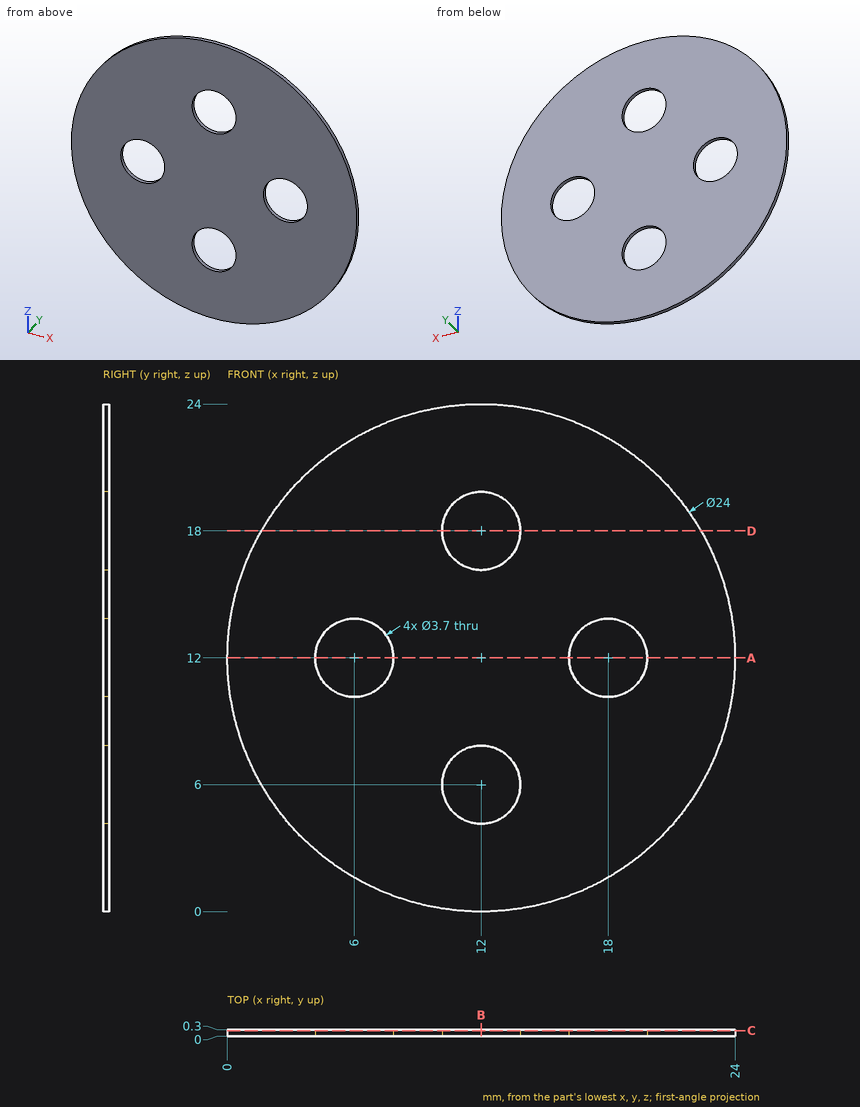
Answer from the drawing. Dimensions are ordinates in mm from the lowest x, y and z of the part. Round coordinates to 2 decimals unless told otherwise and drop trailing zeros. Write each loop counter-clockwise with the first axis right and the second up, starting at its lowest first coordinate (ties: lowest second). Pieces come first, ordered by that corner, then holes. Notation, with made-up numbers: (84.5, 13) - (129.5, 13) arc R32 cw to (129.5, 39) - close; hole circle Ø7 at (-18.75, -21.5). An arc over 180 degrees is marked (long way). One line per item, written item: value.
Q1. Find section D-D (z = 18). Determine the outline of the cut face in (x, y).
The answers:
outline: (1.61, 0) - (10.15, 0) - (10.15, 0.3) - (1.61, 0.3) - close; (13.85, 0) - (22.39, 0) - (22.39, 0.3) - (13.85, 0.3) - close
Q2. Find section B-B (x = 12). Determine the outline of the cut face in (y, z), and give its area (3 significant figures).
The answers:
outline: (0, 0) - (0.3, 0) - (0.3, 4.15) - (0, 4.15) - close; (0, 7.85) - (0.3, 7.85) - (0.3, 16.15) - (0, 16.15) - close; (0, 19.85) - (0.3, 19.85) - (0.3, 24) - (0, 24) - close
area: 4.98 mm2
Q3. Straight lines are drawn through the part: line 1 (X direction, y = 0.1, z = 13); line 2 (Z direction, x = 4.5, y = 0.1); line 3 (Z direction, x = 6, y = 0.1). For each, find the intervals that lie inside material, in ascending order. Write a range as from..to.
The answers:
line 1: x = 0.04..4.44, 7.56..16.44, 19.56..23.96
line 2: z = 2.63..10.92, 13.08..21.37
line 3: z = 1.61..10.15, 13.85..22.39
Q4. Find section C-C (y = 0.25). Determine the outline of the cut face in (x, z), and give its area (3 significant figures).
The answers:
outline: circle Ø24 at (12, 12); hole circle Ø3.7 at (6, 12); hole circle Ø3.7 at (12, 6); hole circle Ø3.7 at (12, 18); hole circle Ø3.7 at (18, 12)
area: 409 mm2
Q5. This flat-tipped pin is pushed along its axis until it touches: P1, Ø3, axis at x = 12, z = 18, coming from the +Y side. Where does it stop, or does it pass through?
The answers:
P1: passes through
Q6. Find section A-A (z = 12). Determine the outline of the cut face in (x, y).
The answers:
outline: (0, 0) - (4.15, 0) - (4.15, 0.3) - (0, 0.3) - close; (7.85, 0) - (16.15, 0) - (16.15, 0.3) - (7.85, 0.3) - close; (19.85, 0) - (24, 0) - (24, 0.3) - (19.85, 0.3) - close
